Part model, mm, in its own coordinate system. Face numbers are marked on the shaded views. A direction names the side the tool comes from. Round coordinates to 2 decimals unless told otherwise and drop trailing zeros. Loops run counter-clockwise (first coordinate to the right, second up) from the corner with the lowest first, then second, coordinate; pieces in that order, holes last. Notation, with made-up numbers: M 2,-10 L 15,-10 A20 ccw 15,14 Z; hole C 20,53.25 d3. An arc over 180 degrees is marked long. Put each result on its own line as item: value. Start each with the question number.
1) Which spindle directions (+Z, -Z, +X, -X, +Y, -Y) get a long thin tool onto all of the face, cutting with end or side? Do the marked faces 1 and 2. Say none if no direction does.
2) Slice it at A-A on y = 1.5. Give the cut face in (x, z), then the cut area to 3 significant figures.
3) Pull direction X, two halves, no side cores. Call the marked faces 3, 4 and 5: +X half, -X half, draft (parallel to the pull), parting line (faces both ways), or undercut.
4) Probe line 1 along Y through (x, z) = (2.25, -2.25); line 2 along X through (y, z) = (11.5, 0); line 3 along Z through (x, y) = (-1.25, 10.75). List the from-to ranges inside material, lowest first.
5) Drop flat-ended pins along their axis: pin 1 Ø1 at (y, z) = (2, -0.5) entering from -X; pin 2 Ø1 at (x, y) = (-1.5, 6.5) entering from +Z; pin 3 Ø4 at (y, z) = (7, -2) entering from +X. Give the stop position or say it passes through.
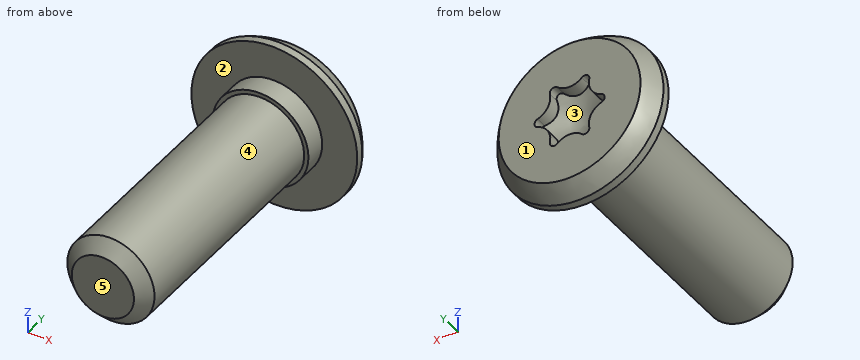
Autodesk Inventor part; units mm, degrees
ref_plane "YZ Plane" through (0, 0, 0) normal (1, 0, 0) x (0, 1, 0)
ref_plane "XZ Plane" through (0, 0, 0) normal (0, 1, 0) x (-1, 0, 0)
ref_plane "XY Plane" through (0, 0, 0) normal (0, 0, 1) x (1, 0, 0)
sketch "Sketch1" plane through (0, 0, 0) normal (0, 1, 0) x (-1, 0, 0)
  circle A0 centre (0, 0) radius 2.0828
  dimension "d4" = 4.1656
extrude "Body" add sketch "Sketch1" along normal blind 12.7
sketch "Sketch2" plane through (0, 0, 0) normal (1, 0, 0) x (0, 1, 0)
  line L0 (12.7, -2.0828) -> (12.7, 2.0828)
  line L1 (12.7, 0) -> (12.7, -3.9624)
  line L2 (12.7, -3.9624) -> (13.081, -3.9624)
  arc A0 (13.081, -3.9624) -> (14.9098, -2.0828) centre (10.8888, 0) ccw
  line L3 (14.9098, -2.0828) -> (14.9098, -1.6764)
  line L4 (14.9098, -1.6764) -> (13.4135, -1.6764)
  line L5 (13.4135, -1.6764) -> (12.8016, 0)
  line L6 (12.8016, 0) -> (12.7, 0)
  point P0 (0, 0)
  dimension "d5" = 3.9624
  dimension "d6" = 0.381
  dimension "d13" = 0.1016
  dimension "d14" = 2.0828
  dimension "d15" = 2.2098
  dimension "d16" = 0
  dimension "d17" = 1.6764
  dimension "d57" = 20.053
revolve "Head" add sketch "Sketch2" angle 360 about axis through (0, 12.8016, 0) along (0, -1, 0)
sketch "Sketch3" plane through (0, 14.9098, 0) normal (0, 1, 0) x (1, 0, 0)
  circle A0 centre (0, 0) radius 1.6764
  line L0 (0.7302, -1.2648) -> (-0.7303, -1.2648) construction
  line L1 (-0.7303, -1.2648) -> (-1.4605, 0) construction
  line L2 (-1.4605, 0) -> (-0.7303, 1.2648) construction
  line L3 (-0.7303, 1.2648) -> (0.7302, 1.2648) construction
  line L4 (0.7302, 1.2648) -> (1.4605, 0) construction
  line L5 (1.4605, 0) -> (0.7302, -1.2648) construction
  circle A1 centre (-0.7303, -1.2648) radius 0.2159
  circle A2 centre (-1.4605, 0) radius 0.2159
  circle A3 centre (-0.7303, 1.2648) radius 0.2159
  circle A4 centre (0.7302, 1.2648) radius 0.2159
  circle A5 centre (1.4605, 0) radius 0.2159
  circle A6 centre (0.7302, -1.2648) radius 0.2159
  circle A7 centre (0, -2.0701) radius 0.8712
  circle A8 centre (0, 2.0701) radius 0.8712
  circle A9 centre (1.7928, -1.0351) radius 0.8712
  circle A10 centre (-1.7928, 1.035) radius 0.8712
  circle A11 centre (1.7928, 1.035) radius 0.8712
  circle A12 centre (-1.7928, -1.0351) radius 0.8712
  circle A13 centre (0, 0) radius 1.8188
  point P0 (0, 0)
  point P1 (0, 0)
  point P2 (0.9413, 1.2192)
  point P3 (1.5265, 0.2056)
  point P4 (1.5265, -0.2056)
  point P5 (0.9413, -1.2192)
  point P6 (0.5852, -1.4248)
  point P7 (-0.5852, -1.4248)
  point P8 (-0.9413, -1.2192)
  point P9 (-1.5265, -0.2056)
  point P10 (-1.5265, 0.2056)
  point P11 (-0.9413, 1.2192)
  point P12 (-0.5852, 1.4248)
  point P13 (0.5852, 1.4248)
  dimension "d58" = 2.921
  dimension "d59" = 4.1402
  dimension "d62" = 120
extrude "Hex" add sketch "Sketch3" against normal blind 1.778 contours A5 A11 A0 | A0 A11 A13 A9 | A0 A9 A5 | A11 A0 | A0 A11 A13 | A9 A13 A0 | A0 A9 | A11 A4 A0 | A0 A8 A13 A11 | A9 A13 A7 A0 | A0 A6 A9 | A4 A8 A0 | A0 A7 A6 | A8 A0 | A7 A0 | A0 A8 A13 | A7 A13 A0 | A3 A0 A8 | A7 A0 A1 | A0 A10 A13 A8 | A7 A13 A12 A0 | A3 A10 A0 | A0 A12 A1 | A10 A0 A13 | A13 A12 A0 | A10 A0 | A0 A12 | A10 A0 A12 A13 | A10 A2 A0 | A0 A2 A12
sketch "Sketch4" plane through (0, 0, 0) normal (0, 0, 1) x (1, 0, 0)
  line L0 (-0.7364, 13.9698) -> (-1.6764, 14.9098)
  line L1 (0, 14.9098) -> (-0.7364, 13.9698)
  line L2 (0, -1.9152) -> (0, 11.491)
  line L3 (-1.5265, 14.9098) -> (-1.5265, 13.3638)
  line L4 (-1.5265, 14.9098) -> (-1.5265, 14.9098)
  line L5 (-1.5265, 14.9098) -> (-1.5265, 13.3638)
  line L6 (-1.6764, 14.9098) -> (-1.5265, 14.9098)
  line L7 (-1.6764, 14.9098) -> (0, 14.9098)
  point P0 (0, 0)
  point P1 (-1.6764, 13.4135)
  dimension "d29" = 1.6764
revolve "Head Chamfer" cut sketch "Sketch4" angle 360 about axis through (0, -10, 0) along (0, 1, 0)
feature "Thread" [suppressed]
sketch "Sketch6" plane through (0, 0, 0) normal (0, 0, 1) x (1, 0, 0)
  line L0 (0, 0) -> (-1.4859, 0)
  line L1 (2.0828, 0) -> (-2.0828, 0)
  line L2 (-1.4859, 0) -> (-2.4948, 1.0089)
  line L3 (-2.4948, 1.0089) -> (-2.9651, -1.2188)
  line L4 (-2.9651, -1.2188) -> (-1.4859, -1.2188)
  line L5 (-2.0828, 0) -> (-2.0828, 12.7)
  line L6 (-1.4859, -1.2188) -> (-1.4859, 0)
  line L7 (0, -2.9358) -> (0, 9.083)
  point P0 (-2.0828, 0.5969)
  dimension "d49" = 1.4859
  dimension "d50" = 135
revolve "Tapered End" cut sketch "Sketch6" angle 360 about axis through (0, -10, 0) along (0, 1, 0)
sketch "Sketch8" plane through (0, 0, 0) normal (0, 0, 1) x (1, 0, 0)
  line L0 (-3.9624, 12.7) -> (3.9624, 12.7)
  line L1 (0, 12.7) -> (2.286, 12.7)
  line L2 (2.286, 12.7) -> (2.286, 11.684)
  line L3 (2.286, 11.684) -> (0, 11.684)
  line L4 (0, 11.684) -> (0, 12.7)
  point P0 (0, 0)
  dimension "d69" = 2.286
  dimension "d70" = 1.016
revolve "Shoulder" add sketch "Sketch8" angle 360 about axis through (0, 11.684, 0) along (0, 1, 0)
sketch "Sketch9" plane through (0, 14.9098, 0) normal (0, 1, 0) x (1, 0, 0)
  circle A0 centre (0, 0) radius 5.7238
  point P0 (0, 0)
extrude "Extrusion3" cut sketch "Sketch9" against normal blind 1.016
sketch "Sketch5" plane through (0, 0, 0) normal (1, 0, 0) x (0, 1, 0)
  line L0 (0, -2.0828) -> (12.7, -2.0828)
  line L1 (12.7, 3.9624) -> (12.7, -3.9624)
  line L2 (12.7, -2.0828) -> (12.7, 2.0828)
  line L3 (0.0745, -2.0828) -> (-0.2261, -2.6035)
  line L4 (-0.2261, -2.6035) -> (-0.3253, -2.6035)
  line L5 (-0.3253, -2.6035) -> (-0.626, -2.0828)
  line L6 (0.0686, -2.6035) -> (-0.7252, -2.6035) construction
  line L7 (-0.626, -2.0828) -> (0.0745, -2.0828)
  line L8 (0, -2.0828) -> (12.7, -2.0828)
  point P0 (0, 0)
  dimension "d31" = 30
  dimension "d32" = 60
  dimension "a" = 0.0992
  dimension "d46" = 0.7937
  dimension "d54" = 0.0686
  dimension "d55" = 0.5207
  dimension "d56" = 0.0992
equation "\"d56\" = a"
equation "\"ShoulderLength\" = 1.016"
properties part number "Shoulder Screw 8-32 Shoulder 0.090 Length 0.290" material "VEX Steel"
Recorded:
1. face 1: +Z, -Z, +X, -X, +Y
1. face 2: -Y
2. outline: C 0,0 d4.17
2. area: 13.6 mm2
3. face 3: undercut
3. face 4: parting line
3. face 5: draft
4. line 1: y = 12.7 to 13.89
4. line 2: x = -2.08 to 2.08
4. line 3: z = -1.67 to 1.67
5. pin 1: stops at x = -2.08
5. pin 2: stops at z = 1.83
5. pin 3: stops at x = 2.08
